Check sheet for the modelled part. Datum: model origin and axes. Units: mm. Coordinates: 2 decimals unless noted, no trailing zeros. Loops run counter-clockwise (first coordinate to the right, second up) from the corner with the lowest first, then second, coordinate; pieces in that order, holes last.
Autodesk Inventor part; units mm, degrees
ref_plane "YZ Plane" through (0, 0, 0) normal (1, 0, 0) x (0, 1, 0)
ref_plane "XZ Plane" through (0, 0, 0) normal (0, 1, 0) x (-1, 0, 0)
ref_plane "XY Plane" through (0, 0, 0) normal (0, 0, 1) x (1, 0, 0)
sketch "Sketch1" plane through (0, 0, 0) normal (0, 1, 0) x (-1, 0, 0)
  circle A0 centre (0, 0.9544) radius 24.13
  point P0 (0, 0)
  dimension "d0" = 48.26
extrude "Extrusion1" add sketch "Sketch1" along normal blind 2.54
sketch "Sketch2" plane through (0, 0, 0.9544) normal (0, -1, 0) x (1, 0, 0)
  circle A0 centre (0, 0) radius 24.13
  line L0 (-8.636, 9.3028) -> (8.636, 9.3028)
  line L1 (8.636, 9.3028) -> (8.636, 16.0337)
  line L2 (8.636, 16.0337) -> (-8.636, 16.0337)
  line L3 (-8.636, 16.0337) -> (-8.636, 9.3028)
  line L4 (0, 0) -> (0, 9.3028) construction
  line L5 (0, 9.3028) -> (0, 16.0337) construction
  dimension "d9" = 17.272
  dimension "d10" = 6.731
  dimension "d11" = 9.3027
extrude "Extrusion2" add sketch "Sketch2" along normal blind 0.0003 and the other way blind 2.5403 contours L3 L2 L1 L0
pattern_circular "Circular Pattern1" count 4 over 360 about axis through (0, 0, 0.9544) along (0, 1, 0) of "Extrusion2"
sketch "Sketch3" plane through (0, 0, 0.9544) normal (0, -1, 0) x (1, 0, 0)
  line L0 (8.636, 9.3027) -> (-8.636, 9.3027)
  circle A0 centre (0, 0) radius 24.13
  line L1 (0, 0) -> (15.7154, 15.7154) construction
  line L2 (0, 0) -> (6.7376, 0) construction
  circle A1 centre (15.7154, 15.7154) radius 1.1303
  dimension "d22" = 22.225
  dimension "d23" = 45
  dimension "d24" = 2.2606
hole "Hole1" at (15.7154, 0, 16.6699) direction (0, 1, 0) diameter 2.2606 depth 25.4 tip angle 118
pattern_circular "Circular Pattern2" count 4 over 360 about axis through (0, 0, 0.9544) along (0, 1, 0) of "Hole1"
sketch "Sketch4" plane through (0, -0.0003, 0.9544) normal (0, -1, 0) x (1, 0, 0)
  line L0 (-8.636, 9.3027) -> (8.636, 9.3027)
  circle A0 centre (0, 12.2237) radius 1.7579
  point P0 (0, -0.9544)
  dimension "d35" = 2.921
hole "Hole2" at (0, -0.0003, 13.1782) direction (0, 1, 0) diameter 4.2926 depth 25.4 tip angle 118
sketch "Sketch5" plane through (0, -0.0003, 0.9544) normal (0, -1, 0) x (1, 0, 0)
  circle A0 centre (0, 12.2237) radius 2.1463
  line L0 (8.636, 16.0337) -> (-8.636, 16.0337)
  circle A1 centre (-6.35, 12.2237) radius 1.1799
  line L1 (0, 12.2237) -> (0, 16.0337) construction
  circle A2 centre (6.35, 12.2237) radius 1.1799
  point P0 (0, -0.9544)
  dimension "d60" = 6.35
hole "Hole3" at (-6.35, -0.0003, 13.1782) at (6.35, -0.0003, 13.1782) direction (0, 1, 0) diameter 2.54 depth 25.4 tip angle 118
pattern_circular "Circular Pattern3" count 4 over 360 about axis through (0, 0, 0.9544) along (0, 1, 0) of "Hole3", "Hole2"
sketch "Sketch6" plane through (0, 2.54, 0.9544) normal (0, 1, 0) x (1, 0, 0)
  line L0 (8.636, -16.0337) -> (-8.636, -16.0337)
  circle A0 centre (0, 0) radius 24.13
  line L1 (0, 24.13) -> (0, 20.828) construction
  line L2 (0, 24.13) -> (3.3047, 20.8253)
  line L3 (0, 24.13) -> (4.6736, 24.13) construction
  line L4 (0, 24.13) -> (-3.3047, 20.8253)
  line L5 (-3.3047, 20.8253) -> (3.3047, 20.8253)
  point P0 (0, 0.9544)
  dimension "d55" = 3.302
  dimension "d56" = 4.6736
  dimension "d57" = 45
extrude "Extrusion3" add sketch "Sketch6" along normal blind 0.0003 contours L2 L5 L4
sketch "Sketch7" plane through (0, 2.54, 0) normal (0, 1, 0) x (1, 0, 0)
  circle A0 centre (0, -0.9544) radius 24.13
  circle A1 centre (0, -0.9544) radius 6.35
  point P0 (0, 0)
  dimension "d61" = 12.7
hole "Hole4" at (0, 2.54, 0.9544) direction (0, -1, 0) diameter 12.7 depth 25.4 tip angle 118
sketch "Sketch8" plane through (9.3027, -0.0003, -7.6816) normal (0, -1, 0) x (1, 0, 0)
  circle A0 centre (2.921, 8.636) radius 2.1463
sketch "Sketch9" plane through (-16.0337, -0.0003, 9.5904) normal (0, -1, 0) x (1, 0, 0)
  circle A0 centre (3.81, -8.636) radius 2.1463
sketch "Sketch10" plane through (0, -0.0003, 0.9544) normal (0, -1, 0) x (1, 0, 0)
  circle A0 centre (0, 12.2237) radius 2.1463
sketch "Sketch11" plane through (-8.636, -0.0003, -8.3483) normal (0, -1, 0) x (1, 0, 0)
  circle A0 centre (8.636, -2.921) radius 2.1463
properties part number "matingBoard"
1) Scan lines: line 1 (X direction, y = 0.6, z = 16.5); line 2 (Z direction, x = -16, y = 1.55); line 3 (X direction, y = 2.3, z = 14). Record each from-to range of solid material in increasing order.
Answer sheet:
line 1: x = -18.46 to -16.83, -14.6 to 14.6, 16.83 to 18.46
line 2: z = -17.11 to -15.85, -13.67 to 15.58, 17.76 to 19.02
line 3: x = -20.3 to -7.32, -5.38 to -1.98, 1.98 to 5.38, 7.32 to 20.3
2) Mould release check, pull along Z, two halves, no side actions. Record for faces 1 (the flat face through (-13.5, 2.54, -1.1)), 2 (the cylindrical face through (15.961, 1.288, -15.864)): +Z half, -Z half, draft (parallel to the pull), parting line (faces both ways), or undercut.
Answer sheet:
face 1: draft
face 2: undercut
3) Section check A-A on x = -12. Give the number of separate pieces and of enclosed holes in the cut face, plus the area to 3 significant figures.
Answer sheet:
separate pieces: 4
enclosed holes: 0
area: 82.8 mm2
4) Section check C-C on z = -18. Enter the section's corners in (x, y).
Answer sheet:
outline: (-14.93, 0) - (14.93, 0) - (14.93, 2.54) - (-14.93, 2.54) - close
5) Depth check by flat-ended pin: pin 1 (4 mm diameter, centred on x = 12.22, z = 0.95, fed in from -Y). Enter the tip coordinate at first touch or a pass-through.
Answer sheet:
pin 1: passes through
6) Section check D-D on x = -21. Enter the section's corners in (y, z).
Answer sheet:
outline: (0, -10.93) - (2.54, -10.93) - (2.54, 12.84) - (0, 12.84) - close
